Source: CAD feature listing. Evaluate the final solid. Frame: model axes, mm. Face numbers are marked on the shaded views. A direction names the side the tool comes from. Coordinates: 2 decimals unless noted, no trailing zeros. Order: outer loops, then holes, each group sorted by start corner. A loop starts at its lowest first (then second) coordinate and runs counter-clockwise, first axis right, second up. Notation, with made-up numbers: (17.25, 31) -> (37.25, 31) arc R21 ccw to (37.25, 42) -> close; hole circle Ø2 at (70, 5.25). An arc over 180 degrees is marked (long way). Write item = value, one per line. Start each with the question number.
Item 1: Section query C-C (x = 54). Output: boundary loops of the cut face in (y, z), then the cut area to 3 significant figures.
Item 2: Section query B-B (x = -10). Output: boundary loops of the cut face in (y, z).
Item 3: Ray query, line 1 along Y through (x, z) = (52, 0); line 2 along Y through (x, z) = (11, 22); line 3 along Y through (x, z) = (14.5, -30). Return the intervals inside material, ascending. Write a range as [from, to].
Item 4: Set-up query: the marked faces 4, 5 and 6. Return all of +Z, -Z, +X, -X, +Y, -Y with unobstructed straight access to the full face (end or side cutting, diameter ignored); none if empty.
Item 5: Mould query, pull axis Y, two halves, no side actions, for the marked faces 1, 2 and 3. Classes: released by +Y, released by -Y, zero draft, split by the parting line, or undercut.
Item 6: Contact query for flat-ended pins moving along their axis: pin 1 (1.6 mm diameter, centred on x = 3.5, y = 30, fed in from +Z); pin 2 (1.6 mm diameter, centred on x = 20, y = -31.5, fed in from -Z); pin 3 (8 mm diameter, centred on x = 2.5, z = -20, fed in from +Y). Output: stop coordinate, or through.
Item 7: Section query A-A (x = 30). Output: boundary loops of the cut face in (y, z).
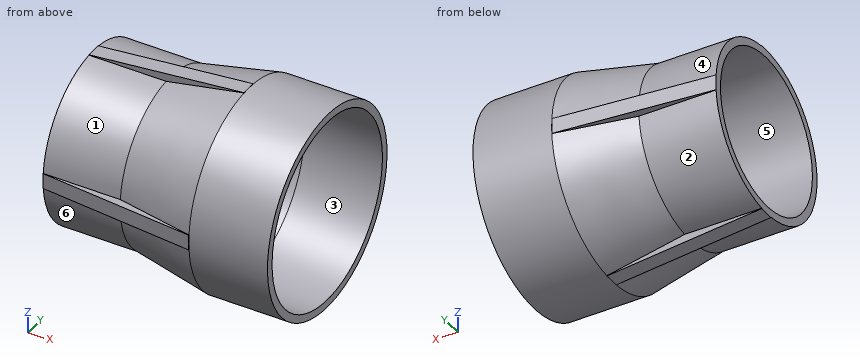
```python
from build123d import *

# Parameters (mm, degrees)
F3_DEPTH = 2.54
F4_COUNT = 4


with BuildPart() as f1:
    # F0 (on Front) → F1 (revolve)
    with BuildSketch(Plane.XZ):
        Polygon((-15.9417227864, 25.4), (9.4582772136, 25.4), (34.8582772136, 30.48), (60.2582772136, 30.48), (60.2582772136, 33.02), (34.606767649, 33.02), (9.206767649, 27.94), (-15.9417227864, 27.94), align=None)
    revolve(axis=Axis((9.6230469644, 0, 0), (-1, 0, 0)))

    # F2 (on Front) → F3 (join, symmetric)
    with BuildSketch(Plane.XZ):
        Polygon((-15.9417227864, 26.67), (9.3325224313, 26.67), (34.8202880916, 31.767553132), (34.5712205999, 33.0128905902), (-15.9417227864, 27.94), align=None)
    extrude(amount=F3_DEPTH, both=True)

    # F4: F1 ×4 about axis
    f4_axis = Axis((9.6230469644, 0, 0), (-1, 0, 0))


with BuildPart() as f1_1:
    add(f1.part)
    for i in range(1, F4_COUNT):
        add(f1.part.rotate(f4_axis, i * 360 / F4_COUNT))


solid = f1_1.part
```
Computed:
q1.outline = circle Ø66.04 at (0, 0); hole circle Ø60.96 at (0, 0)
q1.area = 507 mm^2
q2.outline = (-28.54, -2.54) -> (-27.82, -2.54) arc R27.94 ccw to (-2.54, -27.82) -> (-2.54, -28.54) -> (2.54, -28.54) -> (2.54, -27.82) arc R27.94 ccw to (27.82, -2.54) -> (28.54, -2.54) -> (28.54, 2.54) -> (27.82, 2.54) arc R27.94 ccw to (2.54, 27.82) -> (2.54, 28.54) -> (-2.54, 28.54) -> (-2.54, 27.82) arc R27.94 ccw to (-27.82, 2.54) -> (-28.54, 2.54) -> close; hole circle Ø50.8 at (0, 0)
q3.line_1 = [-33.02, -30.48], [30.48, 33.02]
q3.line_2 = [-17.8, -13.3], [13.3, 17.8]
q3.line_3 = [-2.54, 2.54]
q4.face_4 = +Z, -X, +Y
q4.face_5 = +X, -X
q4.face_6 = -Z, -X, -Y
q5.face_1 = released by -Y
q5.face_2 = released by +Y
q5.face_3 = undercut
q6.pin_1 = 2.54
q6.pin_2 = -2.54
q6.pin_3 = 22.91
q7.outline = (-32.55, -2.54) -> (-32, -2.54) arc R32.1 ccw to (-2.54, -32) -> (-2.54, -32.55) -> (2.54, -32.55) -> (2.54, -32) arc R32.1 ccw to (32, -2.54) -> (32.55, -2.54) -> (32.55, 2.54) -> (32, 2.54) arc R32.1 ccw to (2.54, 32) -> (2.54, 32.55) -> (-2.54, 32.55) -> (-2.54, 32) arc R32.1 ccw to (-32, 2.54) -> (-32.55, 2.54) -> close; hole circle Ø59.02 at (0, 0)
